Can you work these out from the model? Positions are in its coordinate system, mm. A direction names the side the tool comes from. Round coordinates to 2 decimals unless told otherwise and drop trailing zeros. Order: outer loops, then holes, each group sorted by start corner. A loop starts at its lowest first (then second) coordinate and runs counter-clockwise, first axis right, second up.
Q1. For faces 1 (the face through (0, -6, 3)), 2 (the face through (-17.425, -8.479, 12.399)), 3 (the face through (9.946, 3.072, 1.521)), 4 (the face through (10.32, -7.99, 10.22)), which set-ups out of +Z, -Z, +X, -X, +Y, -Y let a thin tool reach every point of the face, with its end or its side?
Q2. If we section it at A-A (y = 0): Please give me the cut outline in (x, z) (3 decimals).
Q3. If we section it at B-B (z = 2.5): Please give me the cut outline in (x, y) (3 decimals), plus the area to 3 significant figures.
Q4. We'd pull the mould along Z, two halves only. Please class faces 5 (the face through (-12.894, -7.986, 5.76)), 6 (the face through (-9.05, -8, 8)), 7 (the face through (0, -10, 6)), 8 (the face through (0, -8, 13)): pulls with the +Z half, pulls with the -Z half, needs draft (parallel to the pull), parting line crosses it, or undercut.
Q5. If I drill on line 1 (X direction, y = -9.6, z = 8) (3 decimals); line 2 (X direction, y = -6.5, z = 3.25) (3 decimals); line 3 (Z direction, x = -14, y = -4.25), over which ranges is the centre line in solid material (lowest first)?
Q6. If we section it at C-C (y = -7.75): Please give me the cut outline in (x, z) (3 decimals).
Q7. If we section it at D-D (y = -2.5): Please give me the cut outline in (x, z) (3 decimals).
Q8. Will these pins go through, and if not, where does the flat tip stop? P1, Ø1.5, axis at x = -1.5, z = 2, coming from the +Y side; P2, Ø3, axis at x = -6, z = 7, coming from the +Y side.
from build123d import *

# Parameters (mm, degrees)
BOSS_EXTRUDE1_DEPTH      = 3
SKETCH2_W                = 35.99
SKETCH2_H                = 3
BOSS_EXTRUDE2_DEPTH      = 13
F_4_CLEARANCE_HOLE1_D    = 3.2639
M2_5X0_45_TAPPED_HOLE1_D = 2.05
CUT_EXTRUDE1_DEPTH       = 25.557484093
CUT_EXTRUDE1_DEPTH_BACK  = 2
FILLET1_R                = 2
RIB1_REACH               = 41.551
SKETCH8_WALL_W           = 87.101962048
SKETCH8_WALL_H           = 1.925
FILLET2_R                = 1.5


with BuildPart() as part:
    # Sketch1 → Boss-Extrude1 (new body)
    with BuildSketch(Plane.XY):
        Polygon((-17.995, 3.5), (-17.995, 0), (-17.995, -10), (17.995, -10), (17.995, 0), (17.995, 3.5), (9.495, 3.5), (9.495, 0), (9.495, -5.5), (-9.495, -5.5), (-9.495, 0), (-9.495, 3.5), align=None)
    extrude(amount=BOSS_EXTRUDE1_DEPTH)

    # Sketch2 → Boss-Extrude2 (add)
    with BuildSketch(Plane.XY):
        with Locations((0, -8.5)):
            Rectangle(SKETCH2_W, SKETCH2_H)
    extrude(amount=BOSS_EXTRUDE2_DEPTH)

    # #4 Clearance Hole1 (through all)
    with Locations(Plane(origin=(0, 0, 0), x_dir=(-1, 0, 0), z_dir=(0, 0, -1))):
        with Locations((12.495, 0), (-12.495, 0)):
            Hole(F_4_CLEARANCE_HOLE1_D / 2)

    # M2.5x0.45 Tapped Hole1 (through all)
    with Locations(Plane(origin=(0, -7, 0), x_dir=(1, 0, 0), z_dir=(0, 1, 0))):
        with Locations((-11.625, -8), (11.625, -8)):
            Hole(M2_5X0_45_TAPPED_HOLE1_D / 2)

    # Sketch9 → Cut-Extrude1 (cut, two sides)
    with BuildSketch(Plane(origin=(0, -7, 0), x_dir=(1, 0, 0), z_dir=(0, 1, 0))) as cut_extrude1_sk:
        Polygon((-9.05, -6.513323057), (-11.625, -5.026646114), (-14.2, -6.513323057), (-14.2, -9.486676943), (-11.625, -10.973353886), (-9.05, -9.486676943), align=None)
        Polygon((11.625, -5.026646114), (9.05, -6.513323057), (9.05, -9.486676943), (11.625, -10.973353886), (14.2, -9.486676943), (14.2, -6.513323057), align=None)
    extrude(amount=CUT_EXTRUDE1_DEPTH, mode=Mode.SUBTRACT)
    extrude(cut_extrude1_sk.sketch, amount=-CUT_EXTRUDE1_DEPTH_BACK, mode=Mode.SUBTRACT)

    # Fillet1
    fillet1_edges = [part.edges().sort_by_distance(p)[0] for p in [
        (-17.995, -8.5, 13),
        (17.995, -8.5, 13),
    ]]
    fillet(fillet1_edges, radius=FILLET1_R)

    # Sketch8 wall → Rib1 (add, up to next)
    with BuildSketch(Plane(origin=(-17.995, -5.5, 5.598076211), x_dir=(0, -0.499999999979, 0.866025403797), z_dir=(0, 0.866025403797, 0.499999999979)), mode=Mode.PRIVATE) as rib1_sk1:
        with Locations((0, 0.9625)):
            Rectangle(SKETCH8_WALL_W, SKETCH8_WALL_H)
    rib1_tool1 = extrude(rib1_sk1.sketch, amount=-RIB1_REACH, mode=Mode.PRIVATE) - part.part
    rib1 = rib1_tool1.solids().sort_by_distance((-17.995, -5.5, 5.598076211))[0]
    add(rib1)

    # Mirror1: Rib1 across plane
    add(rib1.mirror(Plane(origin=(0, 0, 0), x_dir=(0, 0, 1), z_dir=(1, 0, 0))))

    # Fillet2
    fillet2_edges = [part.edges().sort_by_distance(p)[0] for p in [
        (9.495, 3.5, 1.5),
        (9.495, -5.5, 1.5),
        (-9.495, -5.5, 1.5),
        (-9.495, 3.5, 1.5),
        (-17.995, 3.5, 1.5),
        (17.995, 3.5, 1.5),
    ]]
    fillet(fillet2_edges, radius=FILLET2_R)


solid = part.part
Solution:
1. face 1: +Z, +Y
1. face 2: +Z, -X, +Y, -Y
1. face 3: +Z, -Z, +Y
1. face 4: +Y
2. outline: (-17.995, 0) - (-14.127, 0) - (-14.127, 3) - (-17.995, 3) - close; (-10.863, 0) - (-9.495, 0) - (-9.495, 3) - (-10.863, 3) - close; (9.495, 0) - (10.863, 0) - (10.863, 3) - (9.495, 3) - close; (14.127, 0) - (17.995, 0) - (17.995, 3) - (14.127, 3) - close
3. outline: (-17.995, -10) - (17.995, -10) - (17.995, 2) arc R1.5 ccw to (16.495, 3.5) - (10.995, 3.5) arc R1.5 ccw to (9.495, 2) - (9.495, -4) arc R1.5 cw to (7.995, -5.5) - (-7.995, -5.5) arc R1.5 cw to (-9.495, -4) - (-9.495, 2) arc R1.5 ccw to (-10.995, 3.5) - (-16.495, 3.5) arc R1.5 ccw to (-17.995, 2) - close; hole circle Ø3.264 at (-12.495, 0); hole circle Ø3.264 at (12.495, 0)
3. area: 297 mm2
4. face 5: undercut
4. face 6: undercut
4. face 7: needs draft
4. face 8: pulls with the +Z half
5. line 1: x = -17.995 to -12.65, -10.6 to 10.6, 12.65 to 17.995
5. line 2: x = -17.995 to -16.07, 16.07 to 17.995
5. line 3: z = 0 to 3
6. outline: (-17.995, 0) - (17.995, 0) - (17.995, 11) arc R2 ccw to (15.995, 13) - (-15.995, 13) arc R2 ccw to (-17.995, 11) - close; hole (-14.2, 6.513) - (-11.625, 5.027) - (-9.05, 6.513) - (-9.05, 9.487) - (-11.625, 10.973) - (-14.2, 9.487) - close; hole (9.05, 6.513) - (11.625, 5.027) - (14.2, 6.513) - (14.2, 9.487) - (11.625, 10.973) - (9.05, 9.487) - close
7. outline: (-17.995, 0) - (-9.495, 0) - (-9.495, 3) - (-17.995, 3) - close; (9.495, 0) - (17.995, 0) - (17.995, 3) - (9.495, 3) - close
8. P1: stops at y = -5.5
8. P2: stops at y = -7
